Check sheet for the modelled part. Datum: model origin and axes. Units: mm. A direction names the side the tool comes from. Round coordinates to 2 decimals unless told otherwise and drop trailing zeros. Write each loop counter-clockwise with the first axis right and the second up, starting at its lowest first coordinate (ties: lowest second). Pieces come first, ordered by that corner, then holes.
Item 1: Cross-section at D-D on y = -10. Enter the section's corners in (x, z).
Item 2: Cross-section at A-A on y = 22.5. Enter the section's corners in (x, z), plus the area to 3 significant figures.
Item 3: Go/stop test with flat-tipped pins: pin 1 Ø12 at (x, y) = (24.5, -15) entering from +Z; pin 2 Ø1.5 at (y, z) = (26, 2.5) entering from +X; pin 3 Ø3 at (x, z) = (22, 2.5) entering from +Y; pin 4 Ø3 at (x, z) = (-25, 2) entering from -Y. Record where each tip stops, or that it passes through.
Item 4: Tool access check on faces 1 (the cylindrical face through (16.209, 32.194, 3.451)), 2 (the cylindrical face through (-35.985, -2.06, 3.451)). Record the directions out of +Z, -Z, +X, -X, +Y, -Y that give a thin tool (end or side, any length) a straight path to the whole face; none if there is none.
Item 5: Cross-section at B-B on z = 4. Count the separate pieces of the cut face and the enclosed holes in it, plus the area to 3 significant figures.
Item 6: Cross-section at C-C on x = 12. Enter the section's corners in (y, z).
Item 7: Material ranges on line 1 (X direction, y = 24.5, z = 6.75); line 2 (Y direction, x = 18.5, z = 2); line 3 (Y direction, x = -5.5, z = 3), recorded low to high.
from build123d import *

# Parameters (mm, degrees)
F0_R     = 10.65
F1_DEPTH = 7


with BuildPart() as f1:
    # F0 (on Top) → F1 (new body)
    with BuildSketch(Plane.XY):
        with BuildLine():
            ThreePointArc((-13.5850223899, 28.3841313799), (0, 39.0007652062), (13.5850223899, 28.3841313799))
            ThreePointArc((13.5850223899, 28.3841313799), (16.2654595363, 32.2301803319), (20.8939522359, 32.9744189809))
            ThreePointArc((20.8939522359, 32.9744189809), (0, 39.0367717308), (-20.8939522359, 32.9744189809))
            ThreePointArc((-20.8939522359, 32.9744189809), (-16.2654595363, 32.2301803319), (-13.5850223899, 28.3841313799))
        make_face()
        with BuildLine():
            ThreePointArc((-17.7888676444, -25.9570401906), (-33.7756534356, -19.5003826031), (-31.3738900343, -2.4270911893))
            ThreePointArc((-31.3738900343, -2.4270911893), (-36.0448847041, -2.0287890033), (-39.0036606305, 1.6074839313))
            ThreePointArc((-39.0036606305, 1.6074839313), (-33.8068360006, -19.5183858654), (-18.1097083945, -34.5819029122))
            ThreePointArc((-18.1097083945, -34.5819029122), (-19.7794251679, -30.2013913286), (-17.7888676444, -25.9570401906))
        make_face()
        with BuildLine():
            ThreePointArc((39.0036606305, 1.6074839313), (36.0448847041, -2.0287890033), (31.3738900343, -2.4270911893))
            ThreePointArc((31.3738900343, -2.4270911893), (34.537652805, -7.0284675601), (35.6512977827, -12.5003826031))
            ThreePointArc((35.6512977827, -12.5003826031), (30.0752510726, -23.6823775489), (17.7888676444, -25.9570401906))
            ThreePointArc((17.7888676444, -25.9570401906), (19.2622478562, -27.9781893195), (19.783572277, -30.424434176))
            ThreePointArc((19.783572277, -30.424434176), (19.3493973149, -32.6653249916), (18.1097083945, -34.5819029122))
            ThreePointArc((18.1097083945, -34.5819029122), (33.3977102499, -20.2104551465), (39.0367717308, 0))
            ThreePointArc((39.0367717308, 0), (39.0284930779, 0.8039124539), (39.0036606305, 1.6074839313))
        make_face()
        with BuildLine():
            ThreePointArc((-6.3040014892, 12.5003826031), (0, 14), (6.3040014892, 12.5003826031))
            ThreePointArc((6.3040014892, 12.5003826031), (11.832295091, 17.5176647206), (13.9959216435, 24.6628638175))
            ThreePointArc((13.9959216435, 24.6628638175), (13.4927928191, 26.4906281105), (13.5850223899, 28.3841313799))
            ThreePointArc((13.5850223899, 28.3841313799), (0, 39.0007652062), (-13.5850223899, 28.3841313799))
            ThreePointArc((-13.5850223899, 28.3841313799), (-13.4887520947, 27.7699684348), (-13.4565467536, 27.1491408348))
            ThreePointArc((-13.4565467536, 27.1491408348), (-13.592940753, 25.8770855413), (-13.9959216435, 24.6628638175))
            ThreePointArc((-13.9959216435, 24.6628638175), (-11.832295091, 17.5176647206), (-6.3040014892, 12.5003826031))
        make_face()
        with Locations((0, 25.0007652062)):
            Circle(F0_R, mode=Mode.SUBTRACT)
        with BuildLine():
            ThreePointArc((0.5466252979, 11.011440677), (7.9867755981, 7.6001342452), (11.025, 0))
            ThreePointArc((11.025, 0), (10.7168176849, -2.5885215294), (9.8095000075, -5.0323289441))
            ThreePointArc((9.8095000075, -5.0323289441), (11.6657646613, -2.6876802087), (13.9776496359, -0.7907658664))
            ThreePointArc((13.9776496359, -0.7907658664), (13.9944112935, -0.3955408305), (14, 0))
            ThreePointArc((14, 0), (11.9217452759, 7.3397540542), (6.3040014892, 12.5003826031))
            ThreePointArc((6.3040014892, 12.5003826031), (3.5052829927, 11.4466886556), (0.5466252979, 11.011440677))
        make_face()
        with BuildLine():
            ThreePointArc((-9.8095000075, -5.0323289441), (-9.5479300767, 5.5125), (-0.5466252979, 11.011440677))
            ThreePointArc((-0.5466252979, 11.011440677), (-3.5052829927, 11.4466886556), (-6.3040014892, 12.5003826031))
            ThreePointArc((-6.3040014892, 12.5003826031), (-12.124355653, 7), (-13.9776496359, -0.7907658664))
            ThreePointArc((-13.9776496359, -0.7907658664), (-11.6657646613, -2.6876802087), (-9.8095000075, -5.0323289441))
        make_face()
        with BuildLine():
            ThreePointArc((-9.2628747096, -5.9791117329), (-9.5479300767, -5.5125), (-9.8095000075, -5.0323289441))
            ThreePointArc((-9.8095000075, -5.0323289441), (-11.6657646613, -2.6876802087), (-13.9776496359, -0.7907658664))
            ThreePointArc((-13.9776496359, -0.7907658664), (-12.124355653, -7), (-7.6736481467, -11.7096167367))
            ThreePointArc((-7.6736481467, -11.7096167367), (-8.1604816686, -8.7590084469), (-9.2628747096, -5.9791117329))
        make_face()
        with BuildLine():
            ThreePointArc((7.6736481467, -11.7096167367), (8.1604816686, -8.7590084469), (9.2628747096, -5.9791117329))
            ThreePointArc((9.2628747096, -5.9791117329), (0, -11.025), (-9.2628747096, -5.9791117329))
            ThreePointArc((-9.2628747096, -5.9791117329), (-8.1604816686, -8.7590084469), (-7.6736481467, -11.7096167367))
            ThreePointArc((-7.6736481467, -11.7096167367), (0, -14), (7.6736481467, -11.7096167367))
        make_face()
        with BuildLine():
            ThreePointArc((-0.5466252979, 11.011440677), (0, 11.025), (0.5466252979, 11.011440677))
            ThreePointArc((0.5466252979, 11.011440677), (3.5052829927, 11.4466886556), (6.3040014892, 12.5003826031))
            ThreePointArc((6.3040014892, 12.5003826031), (0, 14), (-6.3040014892, 12.5003826031))
            ThreePointArc((-6.3040014892, 12.5003826031), (-3.5052829927, 11.4466886556), (-0.5466252979, 11.011440677))
        make_face()
        with BuildLine():
            ThreePointArc((13.9776496359, -0.7907658664), (11.6657646613, -2.6876802087), (9.8095000075, -5.0323289441))
            ThreePointArc((9.8095000075, -5.0323289441), (9.5479300767, -5.5125), (9.2628747096, -5.9791117329))
            ThreePointArc((9.2628747096, -5.9791117329), (8.1604816686, -8.7590084469), (7.6736481467, -11.7096167367))
            ThreePointArc((7.6736481467, -11.7096167367), (12.124355653, -7), (13.9776496359, -0.7907658664))
        make_face()
        with BuildLine():
            ThreePointArc((28.3566274178, -0.2106082161), (21.0868902085, 1.4882357736), (13.9776496359, -0.7907658664))
            ThreePointArc((13.9776496359, -0.7907658664), (12.124355653, -7), (7.6736481467, -11.7096167367))
            ThreePointArc((7.6736481467, -11.7096167367), (9.2545951175, -19.0059004942), (14.3607057743, -24.4522556014))
            ThreePointArc((14.3607057743, -24.4522556014), (16.1951604964, -24.9304154046), (17.7888676444, -25.9570401906))
            ThreePointArc((17.7888676444, -25.9570401906), (30.0752510726, -23.6823775489), (35.6512977827, -12.5003826031))
            ThreePointArc((35.6512977827, -12.5003826031), (34.537652805, -7.0284675601), (31.3738900343, -2.4270911893))
            ThreePointArc((31.3738900343, -2.4270911893), (29.6879533155, -1.5602127059), (28.3566274178, -0.2106082161))
        make_face()
        with Locations((21.6512977827, -12.5003826031)):
            Circle(F0_R, mode=Mode.SUBTRACT)
        with BuildLine():
            ThreePointArc((-7.6736481467, -11.7096167367), (-12.124355653, -7), (-13.9776496359, -0.7907658664))
            ThreePointArc((-13.9776496359, -0.7907658664), (-21.0868902085, 1.4882357736), (-28.3566274178, -0.2106082161))
            ThreePointArc((-28.3566274178, -0.2106082161), (-29.6879533155, -1.5602127059), (-31.3738900343, -2.4270911893))
            ThreePointArc((-31.3738900343, -2.4270911893), (-33.7756534356, -19.5003826031), (-17.7888676444, -25.9570401906))
            ThreePointArc((-17.7888676444, -25.9570401906), (-16.1951604964, -24.9304154046), (-14.3607057743, -24.4522556014))
            ThreePointArc((-14.3607057743, -24.4522556014), (-9.4433436519, -19.3535465397), (-7.6512977827, -12.5003826031))
            ThreePointArc((-7.6512977827, -12.5003826031), (-7.6568864892, -12.1048417726), (-7.6736481467, -11.7096167367))
        make_face()
        with Locations((-21.6512977827, -12.5003826031)):
            Circle(F0_R, mode=Mode.SUBTRACT)
        with BuildLine():
            ThreePointArc((-31.3738900343, -2.4270911893), (-29.6879533155, -1.5602127059), (-28.3566274178, -0.2106082161))
            ThreePointArc((-28.3566274178, -0.2106082161), (-29.9396844515, -1.2175351599), (-31.3738900343, -2.4270911893))
        make_face()
        with BuildLine():
            ThreePointArc((-13.5850223899, 28.3841313799), (-13.9154258473, 26.5372948962), (-13.9959216435, 24.6628638175))
            ThreePointArc((-13.9959216435, 24.6628638175), (-13.592940753, 25.8770855413), (-13.4565467536, 27.1491408348))
            ThreePointArc((-13.4565467536, 27.1491408348), (-13.4887520947, 27.7699684348), (-13.5850223899, 28.3841313799))
        make_face()
        with BuildLine():
            ThreePointArc((13.5850223899, 28.3841313799), (13.4927928191, 26.4906281105), (13.9959216435, 24.6628638175))
            ThreePointArc((13.9959216435, 24.6628638175), (13.9989803737, 24.8318022062), (14, 25.0007652062))
            ThreePointArc((14, 25.0007652062), (13.8958683331, 26.7051252828), (13.5850223899, 28.3841313799))
        make_face()
        with BuildLine():
            ThreePointArc((31.3738900343, -2.4270911893), (29.9396844515, -1.2175351599), (28.3566274178, -0.2106082161))
            ThreePointArc((28.3566274178, -0.2106082161), (29.6879533155, -1.5602127059), (31.3738900343, -2.4270911893))
        make_face()
        with BuildLine():
            ThreePointArc((17.7888676444, -25.9570401906), (16.1951604964, -24.9304154046), (14.3607057743, -24.4522556014))
            ThreePointArc((14.3607057743, -24.4522556014), (16.0242586042, -25.3197597364), (17.7888676444, -25.9570401906))
        make_face()
        with BuildLine():
            ThreePointArc((-17.7888676444, -25.9570401906), (-16.0242586042, -25.3197597364), (-14.3607057743, -24.4522556014))
            ThreePointArc((-14.3607057743, -24.4522556014), (-16.1951604964, -24.9304154046), (-17.7888676444, -25.9570401906))
        make_face()
    extrude(amount=F1_DEPTH)


solid = f1.part
Response values:
1. outline: (-37.73, 0) - (-32, 0) - (-32, 7) - (-37.73, 7) - close; (-11.3, 0) - (-4.64, 0) - (-4.64, 7) - (-11.3, 7) - close; (4.64, 0) - (11.3, 0) - (11.3, 7) - (4.64, 7) - close; (32, 0) - (37.73, 0) - (37.73, 7) - (32, 7) - close
2. outline: (-13.77, 0) - (-10.35, 0) - (-10.35, 7) - (-13.77, 7) - close; (10.35, 0) - (13.77, 0) - (13.77, 7) - (10.35, 7) - close
2. area: 47.9 mm2
3. pin 1: passes through
3. pin 2: stops at x = 14
3. pin 3: stops at y = 33.22
3. pin 4: stops at y = -31.17
4. face 1: +Z, -Z
4. face 2: +Z, -Z, +Y
5. separate pieces: 1
5. enclosed holes: 4
5. area: 1,220 mm2
6. outline: (-22.64, 0) - (-17, 0) - (-17, 7) - (-22.64, 7) - close; (-8, 0) - (7.21, 0) - (7.21, 7) - (-8, 7) - close; (17.79, 0) - (37.15, 0) - (37.15, 7) - (17.79, 7) - close
7. line 1: x = -13.99 to -10.64, 10.64 to 13.99
7. line 2: y = -34.37 to -34.13, -26.72 to -22.67, -2.33 to 1.14, 33.07 to 34.37
7. line 3: y = -12.87 to -9.56, 9.56 to 15.88, 34.12 to 38.65
